Design review of the part built by this model. Coordinates are the model's own, in mm. A direction names the side the tool comes from. Give positions to 0.01 mm unless a question says otherwise; leave off trailing zeros. Loops run counter-clockwise (first coordinate to the right, second up) from the corner with the lowest first, then second, coordinate; pieces in that order, holes last. Notation, with made-up numbers: M 58,-12 L 114,-12 A34 cw 114,19 Z; hole C 68,73.25 d6. An arc over 180 degrees is marked long. Use CSV: the item, a comma, the result in double quotes.
from build123d import *

# Parameters (mm, degrees)
F0_R     = 28.5304356899
F1_DEPTH = 25.4
F0_W     = 106.1744093895
F0_H     = 18.201328814
F2_DEPTH = 76.2
F4_DEPTH = 18.202328814


with BuildPart() as f1:
    # F0 (on Front) → F1 (new body)
    with BuildSketch(Plane.XZ):
        with BuildLine():
            Line((-53.0872046947, -44.3657338619), (53.0872046947, -44.3657338619))
            Line((53.0872046947, -44.3657338619), (53.0872046947, 5.1191230305))
            ThreePointArc((53.0872046947, 5.1191230305), (0, 58.2063277252), (-53.0872046947, 5.1191230305))
            Line((-53.0872046947, 5.1191230305), (-53.0872046947, -44.3657338619))
        make_face()
        with Locations((0, 5.1191230305)):
            Circle(F0_R, mode=Mode.SUBTRACT)
    extrude(amount=F1_DEPTH)

    # F0 (on Front) → F2 (join)
    with BuildSketch(Plane.XZ):
        with Locations((0, -53.4663982689)):
            Rectangle(F0_W, F0_H)
    extrude(amount=F2_DEPTH)

    # F3 (on face) → F4 (cut, through all)
    with BuildSketch(Plane.XY.offset(-44.3657338619)):
        with BuildLine():
            Line((53.0872046947, -76.2), (53.0872046947, -64.6345680475))
            ThreePointArc((53.0872046947, -64.6345680475), (49.6997681032, -72.8125634085), (41.5217727423, -76.2))
            Line((41.5217727423, -76.2), (53.0872046947, -76.2))
        make_face()
        with BuildLine():
            ThreePointArc((-41.5217727423, -76.2), (-49.6997681032, -72.8125634085), (-53.0872046947, -64.6345680475))
            Line((-53.0872046947, -64.6345680475), (-53.0872046947, -76.2))
            Line((-53.0872046947, -76.2), (-41.5217727423, -76.2))
        make_face()
        Polygon((0, -76.2), (20.6660944968, -76.2), (20.6660944968, -65.4110237956), (-20.6660944968, -65.4110237956), (-20.6660944968, -76.2), align=None)
    extrude(amount=-F4_DEPTH, mode=Mode.SUBTRACT)


solid = f1.part
(1) We need section D-D on z = -30. State the section outline as (x, y) points.
A:
outline,"M -53.09,-25.4 L 53.09,-25.4 L 53.09,0 L -53.09,0 Z"
(2) Clearance check with flat-ended pins moving along their axes: P1, Ø4, axis at x = -10, z = 39.5, coming from the -Y side; P2, Ø5.5, axis at x = 6.5, z = -54, coming from the -Y side; P3, Ø12, axis at y = -73.5, z = -57, coming from the -X side. State where each tip first meets the part, or that it passes through.
A:
P1,"y = -25.4"
P2,"y = -65.41"
P3,"x = -52.73"
(3) We need section A-A on x = 0. State the section outline as (y, z) points, then the cut area to 3 significant figures.
A:
outline,"M -65.41,-62.57 L 0,-62.57 L 0,-23.41 L -25.4,-23.41 L -25.4,-44.37 L -65.41,-44.37 Z; M -25.4,33.65 L 0,33.65 L 0,58.21 L -25.4,58.21 Z"
area,"2,350 mm²"
(4) We need section C-C on x = 15.5. State the section outline as (y, z) points.
A:
outline,"M -65.41,-62.57 L 0,-62.57 L 0,-18.83 L -25.4,-18.83 L -25.4,-44.37 L -65.41,-44.37 Z; M -25.4,29.07 L 0,29.07 L 0,55.89 L -25.4,55.89 Z"
(5) Machinability: for faces 5 (the flat face through (20.666, -71, -53)), 6 (the flat face through (-1, -25.4, -27)), 7 (the flat face through (-31, -76.2, -53)), which of the approach directions +Z, -Z, +X, -X, +Y, -Y give a long, thin tool a straight path to every point of the face, cutting with its end or side? Answer none if there is none.
A:
face 5,"+Z, -Z, -Y"
face 6,"+Z, +X, -X, -Y"
face 7,"+Z, -Z, +X, -X, -Y"
(6) Wall thickness on line 1 along Z through (x, y) = (0, -15.25); line 2 along Y through (x, z) = (12, -47.5); line 3 along Y through (x, z) = (0, -40.5): over which ranges is each line inside the solid? List them lowest first. Write a range as [from, to].
A:
line 1,"[-62.57, -23.41], [33.65, 58.21]"
line 2,"[-65.41, 0]"
line 3,"[-25.4, 0]"
(7) We need section B-B on y = -67. State the section outline as (x, z) points, then the cut area to 3 significant figures.
A:
outline,"M -52.84,-62.57 L -20.67,-62.57 L -20.67,-44.37 L -52.84,-44.37 Z; M 20.67,-62.57 L 52.84,-62.57 L 52.84,-44.37 L 20.67,-44.37 Z"
area,"1,170 mm²"
(8) The part is to be moulded in two halves that separate along X. For faces 1 (the flat face through (-20.666, -71, -53)), 2 (the flat face through (0, -65.411, -53)), 3 (the cylindrical face through (1.167, -12.522, 58.193)), 4 (the flat face through (-1, -50, -44.366)), say which applies: released by +X, released by -X, zero draft, split by the parting line, or undercut.
A:
face 1,"undercut"
face 2,"undercut"
face 3,"split by the parting line"
face 4,"zero draft"
